Answer from the drawing. Dimensions are ordinates in mm from the lowest x, y and z of the part. A direction names the side the tool comes from. Give positions to 0.01 mm unless a question says otherwise; leave off trailing zeros. Loops run counter-clockwise (first coordinate to the right, second up) from the corner with the lowest first, then second, coordinate; pieces in that order, holes last.
(1) Each of these flat-tipped pins is pushed along its axis until it touches: P1, Ø6, axis at y = 11.5, z = 8, coming from the +X side; P2, Ø10, axis at x = 19.5, y = 16, coming from the -Z side; P3, Ø3, axis at x = 20.5, z = 7.5, coming from the +Y side; P4, Ø11, axis at x = 6, z = 15, coming from the +Y side. Where does it stop, or does it pass through?
(2) Find section C-C, the plane y = 20.75. Write down the section's boundary in (x, z), then the cut area to 4 significant figures.
(3) Find section A-A, the plane z = 16.5. Write down the section's boundary in (x, y).
(4) Which of the six approach directions +Z, -Z, +X, -X, +Y, -Y give full straight-line access (tool end or side, diameter ignored) to the marked faces 1, 2 and 3?
(5) Find section B-B, the plane x = 17. Write down the section's boundary in (y, z).
(6) Straight lines are drawn through the part: probe 1 along Z at (x, y) = (9, 17); probe 2 along Y at (x, z) = (10, 6); probe 3 along Y at (x, z) = (36, 21.25). For each, find the intervals that lie inside material, in ascending order.
(7) Find section D-D, the plane x = 42.5. Write down the section's boundary in (y, z).
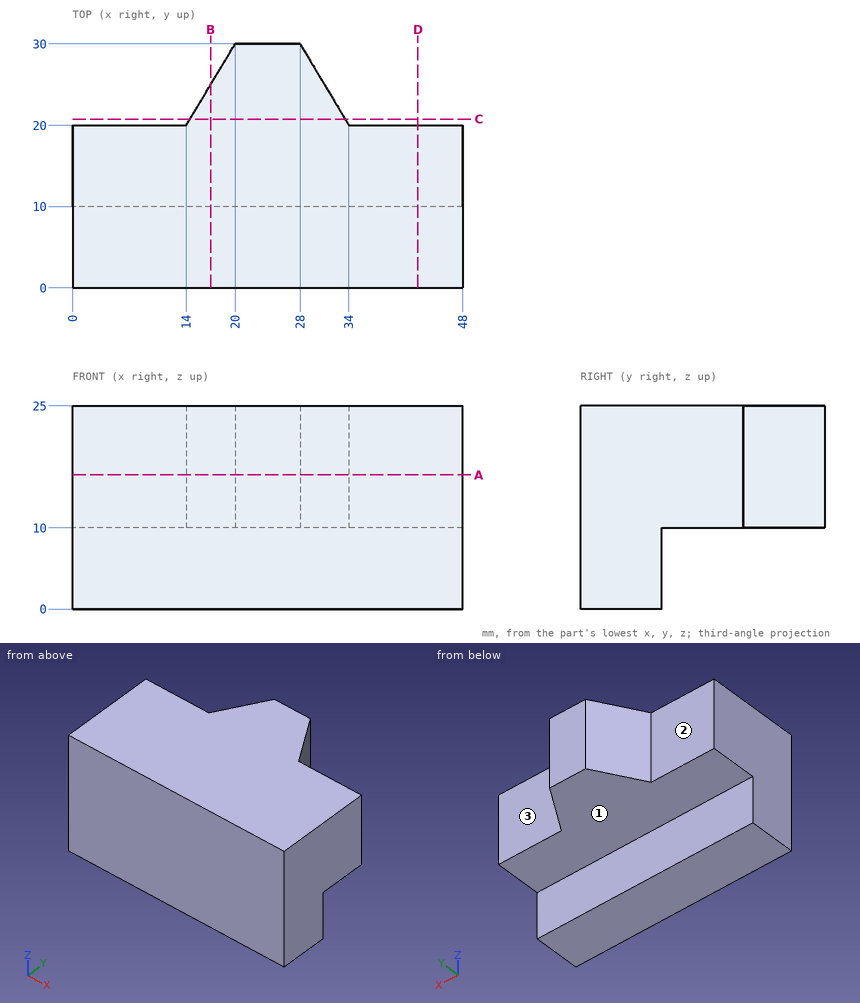
Entries:
1. P1: stops at x = 48
1. P2: stops at z = 10
1. P3: stops at y = 10
1. P4: stops at y = 20
2. outline: (14.45, 10) - (33.55, 10) - (33.55, 25) - (14.45, 25) - close
2. area: 286.5 mm2
3. outline: (0, 0) - (48, 0) - (48, 20) - (34, 20) - (28, 30) - (20, 30) - (14, 20) - (0, 20) - close
4. face 1: -Z, +X, -X, +Y
4. face 2: +Z, -Z, -X, +Y
4. face 3: +Z, -Z, +X, +Y
5. outline: (0, 0) - (10, 0) - (10, 10) - (25, 10) - (25, 25) - (0, 25) - close
6. probe 1: z = 10 to 25
6. probe 2: y = 0 to 10
6. probe 3: y = 0 to 20
7. outline: (0, 0) - (10, 0) - (10, 10) - (20, 10) - (20, 25) - (0, 25) - close
